Could you check a few things on this model? Use its own coordinates, in mm. A direction names the side the tool comes from. Round coordinates to 2 decimals unless told otherwise and drop trailing zeros. Write each loop counter-clockwise with the first axis right and the second up, starting at its lowest first coordinate (ties: lowest second). Pieces come first, ordered by that corner, then holes. Notation, with made-up numbers: (-36, 82) -> (-8, 82) arc R14 ccw to (-8, 97) -> close; hole circle Ø3 at (5, 81). An arc over 180 degrees is marked (long way). One line per question, with ' | ' between items. Start each with the question number.
1. Imagine slicing it at A-A, the plane x = 4.25. List the corners of the cut face in (y, z) for me, and give its area (3 significant figures).
2. For faces 1 (the flat face through (-0.25, 5, 7)), 2 (the flat face through (6, 10, 3)), which set-ups out of +Z, -Z, +X, -X, +Y, -Y let a thin tool reach every point of the face, with its end or its side?
3. Imagine slicing it at B-B, the plane z = 1. List the corners of the cut face in (x, y) for me, and give its area (3 significant figures).
4. Imagine slicing it at C-C, the plane x = 0. List the corners of the cut face in (y, z) for me.
5. Imagine slicing it at D-D, the plane y = 4.25. List the corners of the cut face in (x, z) for me.
6. If I drill on line 1 along X through (y, z) = (9.45, 0); line 2 along X through (y, z) = (5, 0); line 3 along Z through (x, y) = (0, 9.1), over which ranges is the centre line in solid material (lowest first)? Write a range as [from, to].
7. For pin 1 Ø4 at (x, z) = (2, -2) entering from +Y; pin 2 Ø1 at (y, z) = (7, 6) entering from -X; pin 3 Ø2 at (x, y) = (5, 2) entering from -Z; pin 4 Ø1 at (x, y) = (-3, 4) entering from +Z, each with a flat end and sliding along its axis, tell me the tip position at first contact or that it passes through.
8. Thinking about a two-plate mould opening in Z: for faces 3 (the flat face through (-3, 8, -5)), 4 (the flat face through (-1, 0, 6)), which applies, released by +Z, released by -Z, zero draft, split by the parting line, or undercut?
Autodesk Inventor part; units mm, degrees
ref_plane "YZ Plane" through (0, 0, 0) normal (1, 0, 0) x (0, 1, 0)
ref_plane "XZ Plane" through (0, 0, 0) normal (0, 1, 0) x (-1, 0, 0)
ref_plane "XY Plane" through (0, 0, 0) normal (0, 0, 1) x (1, 0, 0)
sketch "スケッチ1" plane through (0, 0, 0) normal (0, 1, 0) x (-1, 0, 0)
  circle A0 centre (0, 0) radius 6.5
  circle A1 centre (0, 0) radius 7.5
  dimension "d0" = 13
  dimension "d11" = 1
extrude "押し出し1" add sketch "スケッチ1" along normal blind 10
sketch "スケッチ2" plane through (0, 0, 0) normal (0, -1, 0) x (1, 0, 0)
  circle A0 centre (0, 0) radius 5.5
  circle A1 centre (0, 0) radius 6.5
  dimension "d12" = 1
extrude "押し出し2" add sketch "スケッチ2" against normal blind 8
sketch "スケッチ3" plane through (0, 10, 0) normal (0, 1, 0) x (1, 0, 0)
  line L0 (0.25, -2.9943) -> (0.25, -7.9943)
  line L1 (0.25, -7.9943) -> (-0.25, -7.9943)
  line L2 (-0.25, -7.9943) -> (-0.25, -2.9943)
  line L3 (-0.25, -2.9943) -> (0, -2.9943)
  line L4 (0, -2.9943) -> (0.25, -2.9943)
  circle A0 centre (0, 0) radius 5.5
  point P0 (0.25, -5.4943)
  dimension "d7" = 0.5
  dimension "d10" = 5
extrude "押し出し3" cut sketch "スケッチ3" against normal through all contours L0 A0 L2 L3 L4 | L0 L1 L2 A0 picked at (-0.1111, -3.8293)
properties part number "zig64"
Geometry results:
1) outline: (0, -6.18) -> (10, -6.18) -> (10, -4.92) -> (8, -4.92) -> (8, -3.49) -> (0, -3.49) -> close; (0, 3.49) -> (8, 3.49) -> (8, 4.92) -> (10, 4.92) -> (10, 6.18) -> (0, 6.18) -> close | area: 48.1 mm2
2) face 1: +Z, +Y, -Y | face 2: +Z, -Z, +X, -X, +Y
3) outline: (-7.43, 0) -> (-5.41, 0) -> (-5.41, 8) -> (-6.42, 8) -> (-6.42, 10) -> (-7.43, 10) -> close; (5.41, 0) -> (7.43, 0) -> (7.43, 10) -> (6.42, 10) -> (6.42, 8) -> (5.41, 8) -> close | area: 36.4 mm2
4) outline: (0, -7.5) -> (10, -7.5) -> (10, -6.5) -> (8, -6.5) -> (8, -5.5) -> (0, -5.5) -> close
5) outline: (-0.25, 5.49) -> (-0.25, 7.5) arc R7.5 ccw (long way) to (0.25, 7.5) -> (0.25, 5.49) arc R5.5 cw (long way) to start
6) line 1: x = [-7.5, -6.5], [6.5, 7.5] | line 2: x = [-7.5, -5.5], [5.5, 7.5] | line 3: z = [-7.5, -6.5]
7) pin 1: passes through | pin 2: stops at x = -5.1 | pin 3: stops at z = -6.34 | pin 4: stops at z = 7.07
8) face 3: undercut | face 4: zero draft
